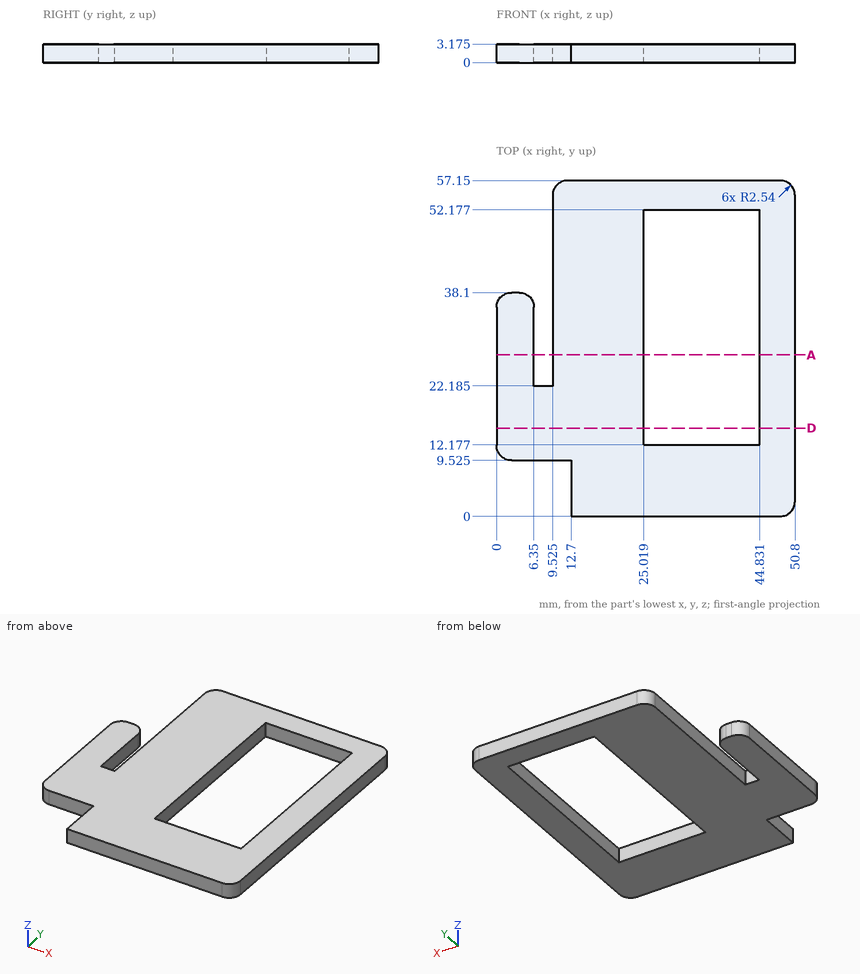
The drawing under review shows one solid part. Ordinate dimensions are in mm from its lowest x, y, z. Give positions to 0.01 mm unless a question says otherwise; leave off trailing zeros. Order: outer loops, then holes, each group sorted by start corner. A loop starts at its lowest first (then second) coordinate and runs counter-clockwise, first axis right, second up. Notation, with made-up numbers: (84.5, 15.5) - (113.5, 15.5) arc R12 cw to (113.5, 25.5) - close; hole circle Ø3 at (62, -20.75). An arc over 180 degrees is marked (long way). Answer as a JSON object with one key per item and string values. Group by question number.
Item 1: Wall thickness on line 1 along X through (y, z) = (31, 2.4) (3 decimals); line 2 along X through (y, z) = (48, 2.45) (3 decimals); line 3 along Y through (x, z) = (30, 1.2): over which ranges is each line inside the solid? List them lowest first.
Item 2: Take a section at A-A on y = 27.5. Give the boundary of the cut face in (x, z) (3 decimals), and give its area (3 significant figures).
Item 3: Take a section at D-D on y = 15. Give the boundary of the cut face in (x, z) (3 decimals), and give its area (3 significant figures).
Item 4: Clearance check with flat-ended pins moving along their axes: pin 1 Ø1 at (x, z) = (3.5, 1) entering from +Y; pin 2 Ø1 at (y, z) = (39.5, 1.5) entering from -X (3 decimals); pin 3 Ø1 at (y, z) = (6, 1) entering from -X. State where each tip first meets the part, or that it passes through.
Reported:
{
 "1": {"line 1": "0 to 6.35, 9.525 to 25.019, 44.831 to 50.8", "line 2": "9.525 to 25.019, 44.831 to 50.8", "line 3": "0 to 12.18, 52.18 to 57.15"},
 "2": {"outline": "(0, 0) - (6.35, 0) - (6.35, 3.175) - (0, 3.175) - close; (9.525, 0) - (25.019, 0) - (25.019, 3.175) - (9.525, 3.175) - close; (44.831, 0) - (50.8, 0) - (50.8, 3.175) - (44.831, 3.175) - close", "area": "88.3 mm^2"},
 "3": {"outline": "(0, 0) - (25.019, 0) - (25.019, 3.175) - (0, 3.175) - close; (44.831, 0) - (50.8, 0) - (50.8, 3.175) - (44.831, 3.175) - close", "area": "98.4 mm^2"},
 "4": {"pin 1": "y = 38.1", "pin 2": "x = 9.525", "pin 3": "x = 12.7"}
}
